The figure shows three views and two pictorial views of one solid part (mm, origin at its lowest corner). Answer the questions. Coordinates: 2 decimals unless noted, no trailing zeros. Loops run counter-clockwise (first coordinate to the right, second up) from the corner with the lowest first, then second, coordinate; pieces in that order, holes last. Notation, with made-up numbers: (41, 25) - (83, 25) arc R25 ccw to (83, 58) - close; hole circle Ø9 at (61, 24). An arc over 180 degrees is marked (long way). Return JSON: item names as keys, results as strings. Group by question number.
1. Section C-C (z = 33.5) is taken. Write down the section's boundary in (x, y), and give its area (3 significant figures).
2. Find the intervals of material crossed by line 1 along Z through (x, y) = (88.5, 2); line 2 along X through (y, z) = (5.5, 20); line 3 along Z through (x, y) = (50, 4.75), in increasing order.
3. Section A-A (x = 50) is taken. Write down the section's boundary in (y, z).
4. Section B-B (y = 2) is taken. Write down the section's boundary in (x, z), and give its area (3 significant figures).
5. Section D-D (z = 20) is taken. Write down the section's boundary in (x, y), and give its area (3 significant figures).
6. This flat-tipped pin is pushed along its axis until it touches: P1, Ø2, axis at x = 27.5, z = 20, coming from the +Y side. Where does it stop, or does it pass through?
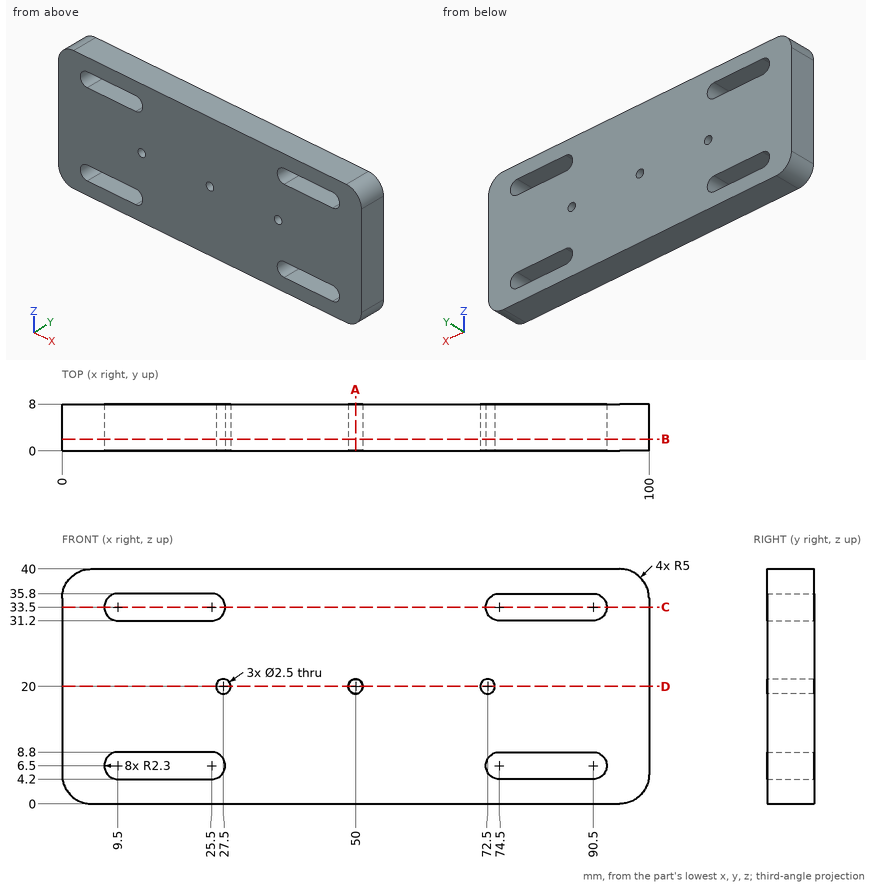
The answers:
{
 "1": {"outline": "(0, 0) - (7.2, 0) - (7.2, 8) - (0, 8) - close; (27.8, 0) - (72.2, 0) - (72.2, 8) - (27.8, 8) - close; (92.8, 0) - (100, 0) - (100, 8) - (92.8, 8) - close", "area": "470 mm2"},
 "2": {"line 1": "z = 0 to 4.2, 8.8 to 31.2, 35.8 to 40", "line 2": "x = 0 to 26.25, 28.75 to 48.75, 51.25 to 71.25, 73.75 to 100", "line 3": "z = 0 to 18.75, 21.25 to 40"},
 "3": {"outline": "(0, 0) - (8, 0) - (8, 18.75) - (0, 18.75) - close; (0, 21.25) - (8, 21.25) - (8, 40) - (0, 40) - close"},
 "4": {"outline": "(0, 5) arc R5 ccw to (5, 0) - (95, 0) arc R5 ccw to (100, 5) - (100, 35) arc R5 ccw to (95, 40) - (5, 40) arc R5 ccw to (0, 35) - close; hole (9.5, 4.2) - (25.5, 4.2) arc R2.3 ccw to (25.5, 8.8) - (9.5, 8.8) arc R2.3 ccw to start; hole (9.5, 31.2) - (25.5, 31.2) arc R2.3 ccw to (25.5, 35.8) - (9.5, 35.8) arc R2.3 ccw to start; hole circle Ø2.5 at (27.5, 20); hole circle Ø2.5 at (50, 20); hole circle Ø2.5 at (72.5, 20); hole (74.5, 4.2) - (90.5, 4.2) arc R2.3 ccw to (90.5, 8.8) - (74.5, 8.8) arc R2.3 ccw to start; hole (74.5, 31.2) - (90.5, 31.2) arc R2.3 ccw to (90.5, 35.8) - (74.5, 35.8) arc R2.3 ccw to start", "area": "3,600 mm2"},
 "5": {"outline": "(0, 0) - (26.25, 0) - (26.25, 8) - (0, 8) - close; (28.75, 0) - (48.75, 0) - (48.75, 8) - (28.75, 8) - close; (51.25, 0) - (71.25, 0) - (71.25, 8) - (51.25, 8) - close; (73.75, 0) - (100, 0) - (100, 8) - (73.75, 8) - close", "area": "740 mm2"},
 "6": {"P1": "passes through"}
}
